Verification items for the finished model (mm, model axes). Face numbers are marked on the shaded views. Round coordinates to 2 decimals unless told otherwise and drop trailing zeros. Write each loop counter-clockwise with the first axis right and the second up, starting at its lowest first coordinate (ties: lowest second). Pieces come first, ordered by that corner, then holes. Notation, with made-up numbers: M 52.25,8 L 92.25,8 A19 ccw 92.25,37 Z; hole C 43,35 d3. An arc over 180 degrees is marked long. Write each question's results on one line, items separated by ' | '.
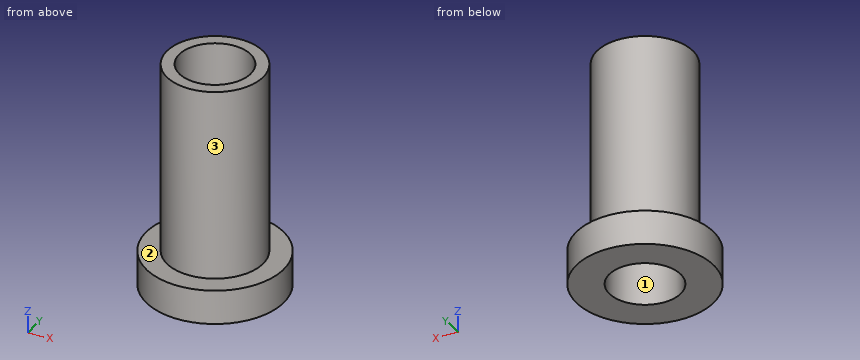
from build123d import *

# Parameters (mm, degrees)
CYLINDER110_R     = 1.5
CYLINDER110_DEPTH = 11
CYLINDER104_R     = 5.2
CYLINDER104_DEPTH = 46
CYLINDER109_R     = 1.5
CYLINDER109_DEPTH = 11
BOX018_W          = 14
BOX018_H          = 1
BOX018_DEPTH      = 5
CYLINDER102_R     = 10
CYLINDER102_DEPTH = 5
CYLINDER071_R     = 7
CYLINDER071_DEPTH = 33


with BuildPart() as obj1:
    # Cylinder110 → Cylinder110 (new body)
    with BuildSketch(Plane(origin=(99.69, 175.69, -10), x_dir=(1, 0, 0), z_dir=(0, 0, 1))):
        Circle(CYLINDER110_R)
    extrude(amount=CYLINDER110_DEPTH)


with BuildPart() as obj2:
    # Cylinder104 → Cylinder104 (new body)
    with BuildSketch(Plane(origin=(86.69, 175.69, -14), x_dir=(1, 0, 0), z_dir=(0, 0, 1))):
        Circle(CYLINDER104_R)
    extrude(amount=CYLINDER104_DEPTH)


with BuildPart() as fusion046:
    # Cylinder109 → Cylinder109 (new body)
    with BuildSketch(Plane(origin=(73.69, 175.69, -10), x_dir=(1, 0, 0), z_dir=(0, 0, 1))):
        Circle(CYLINDER109_R)
    extrude(amount=CYLINDER109_DEPTH)

    # Fusion046: union obj1, obj2
    add(obj1.part)
    add(obj2.part)


with BuildPart() as obj3:
    # Box018 → Box018 (new body)
    with BuildSketch(Plane(origin=(77.69, 171.69, -5), x_dir=(1, 0, 0), z_dir=(0, 0, 1))):
        with Locations((7, 0.5)):
            Rectangle(BOX018_W, BOX018_H)
    extrude(amount=BOX018_DEPTH)


with BuildPart() as obj4:
    # Cylinder102 → Cylinder102 (new body)
    with BuildSketch(Plane(origin=(86.69, 175.69, -5), x_dir=(1, 0, 0), z_dir=(0, 0, 1))):
        Circle(CYLINDER102_R)
    extrude(amount=CYLINDER102_DEPTH)


with BuildPart() as obj5:
    # Cylinder071 → Cylinder071 (new body)
    with BuildSketch(Plane(origin=(86.69, 175.69, -5), x_dir=(1, 0, 0), z_dir=(0, 0, 1))):
        Circle(CYLINDER071_R)
    extrude(amount=CYLINDER071_DEPTH)

    # Fusion045: union obj3, obj4
    add(obj3.part)
    add(obj4.part)

    # Cut013: cut Fusion046
    add(fusion046.part, mode=Mode.SUBTRACT)


solid = obj5.part
1) Sectioned sample at D-D, the plane x = 92.75. Record the cut outline in (y, z).
Calculated:
outline: M 167.74,-5 L 183.64,-5 L 183.64,0 L 179.19,0 L 179.19,28 L 172.19,28 L 172.19,0 L 167.74,0 Z
2) Sectioned sample at A-A, the plane x = 86.69. Record the cut outline in (y, z).
Calculated:
outline: M 165.69,-5 L 170.49,-5 L 170.49,28 L 168.69,28 L 168.69,0 L 165.69,0 Z; M 180.89,-5 L 185.69,-5 L 185.69,0 L 182.69,0 L 182.69,28 L 180.89,28 Z
3) Material ranges on line 1 (Y direction, x = 86.69, z = 18); line 2 (X direction, y = 175.69, z = 10.5); line 3 (X direction, y = 179.25, z = 25.5), recorded low to high. Write a range as [from, to].
Calculated:
line 1: y = [168.69, 170.49], [180.89, 182.69] | line 2: x = [79.69, 81.49], [91.89, 93.69] | line 3: x = [80.66, 82.9], [90.48, 92.72]
4) Depth check by flat-ended pin: P1, Ø5, axis at y = 176.5, z = 21, coming from the -X side; P2, Ø1, axis at x = 85, z = 18.5, coming from the -Y side; P3, Ø8, axis at y = 171, z = 2.5, coming from the -X side. Enter the tip coordinate at first touch or a pass-through.
Calculated:
P1: stops at x = 79.69 | P2: stops at y = 168.79 | P3: stops at x = 76.81
5) Sectioned sample at C-C, the plane z = 5.5. Record the cut outline in (x, y).
Calculated:
outline: C 86.69,175.69 d14; hole C 86.69,175.69 d10.4
6) Draft check along X on the marked faces 1, 2 and 3. Enter one of: pulls with the +X half, pulls with the -X half, needs draft (parallel to the pull), parting line crosses it, or undercut.
Calculated:
face 1: undercut | face 2: needs draft | face 3: parting line crosses it
7) Sectioned sample at B-B, the plane y = 175.69. Record the cut outline in (x, z).
Calculated:
outline: M 76.69,-5 L 81.49,-5 L 81.49,28 L 79.69,28 L 79.69,0 L 76.69,0 Z; M 91.89,-5 L 96.69,-5 L 96.69,0 L 93.69,0 L 93.69,28 L 91.89,28 Z
